Work out the finished part from the listing and answer in its coordinate system (mm). Face numbers are marked on the shaded views. A direction names the side the tool comes from. Round coordinates to 2 decimals unless told otherwise and drop trailing zeros. Loops run counter-clockwise (first coordinate to the right, second up) from the corner with the lowest first, then second, coordinate; pieces in that order, holes last.
```python
from build123d import *

# Parameters (mm, degrees)
SKETCH2_W           = 25.4
SKETCH2_H           = 22.86
BOSS_EXTRUDE1_DEPTH = 2
SKETCH5_R           = 1.27
CUT_EXTRUDE1_DEPTH  = 3
FILLET1_R           = 2.54
SKETCH6_W           = 5.5
SKETCH6_H           = 6
BOSS_EXTRUDE2_DEPTH = 2.9


with BuildPart() as part:
    # Sketch2 → Boss-Extrude1 (new body)
    with BuildSketch(Plane(origin=(0, 0, 0), x_dir=(1, 0, 0), z_dir=(0, 1, 0))):
        with Locations((12.7, 11.43)):
            Rectangle(SKETCH2_W, SKETCH2_H)
    extrude(amount=BOSS_EXTRUDE1_DEPTH)

    # Sketch5 → Cut-Extrude1 (cut, through all)
    with BuildSketch(Plane(origin=(0, 2, 0), x_dir=(1, 0, 0), z_dir=(0, 1, 0))):
        with Locations((2.54, 2.54)):
            Circle(SKETCH5_R)
        with Locations((22.86, 2.54)):
            Circle(SKETCH5_R)
        with Locations((22.86, 20.32)):
            Circle(SKETCH5_R)
        with Locations((2.54, 20.32)):
            Circle(SKETCH5_R)
    extrude(amount=-CUT_EXTRUDE1_DEPTH, mode=Mode.SUBTRACT)

    # Fillet1
    fillet1_edges = [part.edges().sort_by_distance(p)[0] for p in [
        (0, 1, -22.86),
        (25.4, 1, -22.86),
        (25.4, 1, 0),
        (0, 1, 0),
    ]]
    fillet(fillet1_edges, radius=FILLET1_R)

    # Sketch6 → Boss-Extrude2 (add)
    with BuildSketch(Plane(origin=(0, 2, 0), x_dir=(1, 0, 0), z_dir=(0, 1, 0))):
        with Locations((2.75, 11.43)):
            Rectangle(SKETCH6_W, SKETCH6_H)
        with Locations((22.65, 11.43)):
            Rectangle(SKETCH6_W, SKETCH6_H)
    extrude(amount=BOSS_EXTRUDE2_DEPTH)


solid = part.part
```
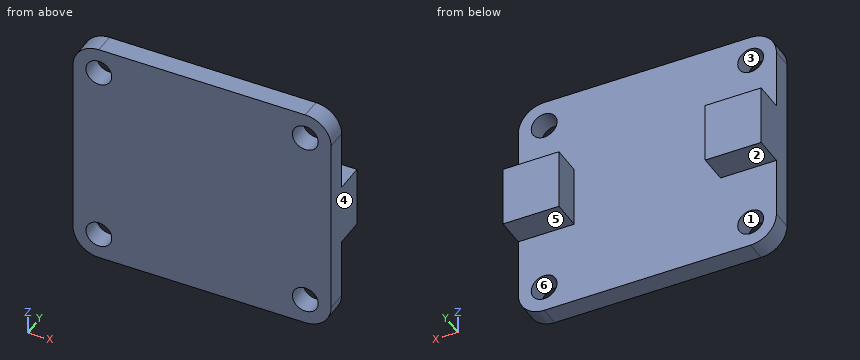
1. Given pin 1 (0.9 mm diameter, centred on x = 22.5, y = 3.5, fed in from -Z); pin 2 (0.9 mm diameter, centred on x = 23, y = 3.5, fed in from +Z); pin 3 (2 mm diameter, centred on x = 20, z = -20, fed in from +Y), each flat-ended and moving along its own axis, determine where each tip first touches the part or whether it passes through.
Answer key:
pin 1: stops at z = -14.43
pin 2: stops at z = -8.43
pin 3: stops at y = 2
2. Find section C-C (x = 4.5). Write down the section's boundary in (y, z).
Answer key:
outline: (0, -22.86) - (2, -22.86) - (2, -14.43) - (4.9, -14.43) - (4.9, -8.43) - (2, -8.43) - (2, 0) - (0, 0) - close
3. Consider probe 1 along Z at (x, y) = (22.86, 1.15); probe 2 along X at (y, z) = (1.55, -20.32); probe 3 along Y at (x, z) = (13, -16). Determine where each line is inside the solid, lowest interval first.
Answer key:
probe 1: z = -22.86 to -21.59, -19.05 to -3.81, -1.27 to 0
probe 2: x = 0 to 1.27, 3.81 to 21.59, 24.13 to 25.4
probe 3: y = 0 to 2
4. Determine the mould class of the marked faces 3, 4, 5 and 6 for opening direction X: +X half, -X half, draft (parallel to the pull), parting line (faces both ways), or undercut.
Answer key:
face 3: undercut
face 4: +X half
face 5: draft
face 6: undercut
5. Find section A-A (y = 2.85). Write down the section's boundary in (x, z).
Answer key:
outline: (0, -14.43) - (5.5, -14.43) - (5.5, -8.43) - (0, -8.43) - close; (19.9, -14.43) - (25.4, -14.43) - (25.4, -8.43) - (19.9, -8.43) - close
6. Which of the six approach directions +Z, -Z, +X, -X, +Y, -Y give full straight-line access (tool end or side, diameter ignored) to the marked faces 1 and 2?
Answer key:
face 1: +Y, -Y
face 2: -Z, +X, -X, +Y
7. Find section B-B (y = 0.6). Write down the section's boundary in (x, z).
Answer key:
outline: (0, -20.32) arc R2.54 ccw to (2.54, -22.86) - (22.86, -22.86) arc R2.54 ccw to (25.4, -20.32) - (25.4, -2.54) arc R2.54 ccw to (22.86, 0) - (2.54, 0) arc R2.54 ccw to (0, -2.54) - close; hole circle Ø2.54 at (2.54, -20.32); hole circle Ø2.54 at (2.54, -2.54); hole circle Ø2.54 at (22.86, -20.32); hole circle Ø2.54 at (22.86, -2.54)
8. Find section D-D (z = -3.25). Write down the section's boundary in (x, y), then the cut area to 3 significant figures.
Answer key:
outline: (0, 0) - (1.49, 0) - (1.49, 2) - (0, 2) - close; (3.59, 0) - (21.81, 0) - (21.81, 2) - (3.59, 2) - close; (23.91, 0) - (25.4, 0) - (25.4, 2) - (23.91, 2) - close
area: 42.4 mm2
